Geometry: see drawing. Coordinates: mm, zero at the bounding-box minimum. A direction names the side the tool comes from. Round coordinates to 2 decimals unless told otherwise and drop trailing zeros. Loops run counter-clockwise (first coordinate to the right, second up) from the corner with the lowest first, then second, coordinate; pieces in that order, holes last.
(1) Cut plane C-C, the plane x = 22.5. Output: boundary loops of the cut face in (y, z).
(2) Cut plane A-A, the plane y = 25. Output: boundary loops of the cut face in (x, z).
(3) Cut plane B-B, the plane z = 16.5. Output: boundary loops of the cut face in (x, y) (1 decimal).
(4) First-contact query: pin 1 Ø12.5 at (y, z) = (61.5, 16.5) entering from +X. Flat tip, straight axial feed; report the tip coordinate or a pass-through.
(5) Cut plane D-D, the plane y = 41. Output: boundary loops of the cut face in (x, z).
(6) Draft query along Z for the marked faces 1, 2 and 3. Return one class per face: released by +Z, released by -Z, zero draft, split by the parting line, or undercut.
(7) Access query for the marked faces 4 and 5. Directions: +Z, -Z, +X, -X, +Y, -Y. A direction counts if a zero-diameter tool reaches every point of the face in a straight line with its end or side. Return the directions, or none.
(8) Line query: line 1 (Z direction, x = 12.5, y = 61); line 2 (Z direction, x = 1.2, y = 120); line 3 (X direction, y = 103.5, z = 7). Output: solid intervals per line, ascending.
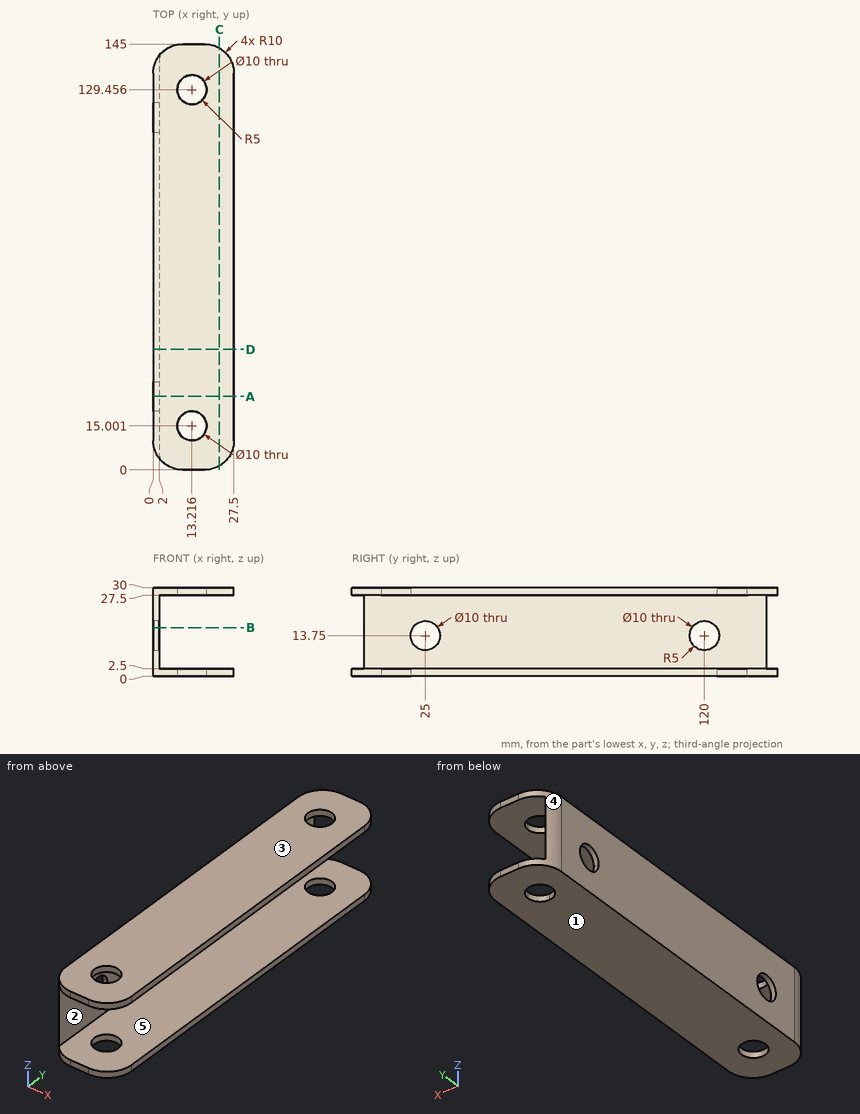
Reported:
1. outline: (1.34, 0) - (143.66, 0) - (143.66, 2.5) - (1.34, 2.5) - close; (1.34, 27.5) - (143.66, 27.5) - (143.66, 30) - (1.34, 30) - close
2. outline: (0, 0) - (27.5, 0) - (27.5, 2.5) - (2, 2.5) - (2, 8.75) - (0, 8.75) - close; (0, 18.75) - (2, 18.75) - (2, 27.5) - (27.5, 27.5) - (27.5, 30) - (0, 30) - close
3. outline: (0, 10) arc R10 ccw to (2, 4) - (2, 20.8) - (0, 20.8) - close; (0, 29.2) - (2, 29.2) - (2, 115.8) - (0, 115.8) - close; (0, 124.2) - (2, 124.2) - (2, 141) arc R10 ccw to (0, 135) - close
4. pin 1: stops at x = 2
5. outline: (0, 0) - (27.5, 0) - (27.5, 2.5) - (2, 2.5) - (2, 27.5) - (27.5, 27.5) - (27.5, 30) - (0, 30) - close
6. face 1: released by -Z
6. face 2: undercut
6. face 3: released by +Z
7. face 4: +Z, -Z, -X, +Y
7. face 5: +X, +Y, -Y
8. line 1: z = 0 to 2.5, 27.5 to 30
8. line 2: z = 0 to 8.75, 18.75 to 30
8. line 3: x = 0 to 2
